The model under review builds one solid part; all positions refer to its coordinate system, in mm. A direction names the side the tool comes from. Round coordinates to 2 decimals unless told otherwise and drop trailing zeros. Order: outer loops, then holes, each group sorted by start corner. A loop starts at its lowest first (then second) coordinate and runs counter-clockwise, first axis right, second up. Notation, with made-up numbers: M -12,-27 L 10,-27 A16 ccw 10,-2 Z; hole C -28.5,38 d4. An arc over 180 degrees is marked long. Use a Markdown table: item, result. Add a question column.
1. The part is to be moulded in two halves that separate along X. For faces 4 (the cylindrical face through (0.04, -4.72, 1.76)), 5 (the cylindrical face through (-0.014, -4.393, -1.511)), say which applies: +X half, -X half, draft (parallel to the pull), parting line (faces both ways), or undercut.
2. Consider section A-A on y = 7. State the section outline as (x, z) points.
3. For faces 1 (the cylindrical face through (-0.108, 6.512, 0.004)), 2 (the flat face through (0.01, -3.3, -0.48)), 3 (the cylindrical face through (-0.192, -4.716, 0.048)), list the 3-axis set-ups (+Z, -Z, +X, -X, +Y, -Y) from which the entire face can be reached by the end or side of a thin tool; tool diameter is ignored.
4. Insertion check: P1, Ø2, axis at x = -2, y = 1.5, coming from the +Z side; P2, Ø1.5, axis at y = 4, z = -0.5, coming from the -X side; P3, Ø0.6, axis at x = -2.5, z = 0, coming from the +Y side. Each pin has a flat end and moves straight along its axis. Give the tip position at first contact, or say it passes through.
5. Consider section B-B on x = 0. State the section outline as (y, z) points.
6. To check wall thickness, follow probe 1 along Z at (x, y) = (-0.25, 5.5); probe 2 along X at (y, z) = (1.75, 0.1); probe 3 along Y at (x, z) = (0.5, 1.55). State the ranges of each line that lie inside material, in increasing order.
7. Consider section D-D on x = -0.75. State the section outline as (y, z) points, then the cut area to 3 significant figures.
8. Consider section C-C on z = 0.7. State the section outline as (x, y) points, then the cut area to 3 significant figures.
from build123d import *

# Parameters (mm, degrees)
MAINBODYS_W                           = 2.8
MAINBODYS_H                           = 0.5
MAIN_BODY_DEPTH                       = 9.5
BOTTOM_OF_MAIN_BODY_REACH             = 11.606
BOTTOM_OF_MAIN_BODY_DIRECTION_2_REACH = 11.606
TOPHOLES_R                            = 0.5
TOP_HOLE_DEPTH                        = 11.069260152
F_45_DEGREE_FLANGE_DEPTH              = 2
BOTTOM_FLAT_FLANGE_DEPTH              = 2
EXTENDEDBOTTOMFLANGES_W               = 2
EXTENDEDBOTTOMFLANGES_H               = 0.5
EXTENDED_BOTTOM_FLANGE_DEPTH          = 0.4
BOSSEDCYLINDERBODYS_R                 = 0.5
BOSSED_CYLINDER_BODY_DEPTH            = 0.5
C_MAIN_BODY_SIZE                      = 0.4


# Sheet-metal steps are written as plain solids
with BuildPart() as part:
    # MainBodyS → MAIN BODY (new body)
    with BuildSketch(Plane(origin=(0, 0, 0), x_dir=(1, 0, 0), z_dir=(0, 1, 0))):
        Rectangle(MAINBODYS_W, MAINBODYS_H)
    extrude(amount=MAIN_BODY_DEPTH)

    # BOTTOM OF MAIN BODY: up to this face of the body (flat: up to its plane)
    bottom_of_main_body_end = Plane(part.part.faces().sort_by_distance((0, 4.75, 0.25))[0])
    # BottomMainBodyS → BOTTOM OF MAIN BODY (add, up to the picked face)
    with BuildSketch(Plane.XY, mode=Mode.PRIVATE) as bottom_of_main_body_sk1:
        Polygon((0, 0), (2.8, 0), (2.8, -2), (3.3, -5), (2.2, -5), (1.2, -2.2), (0, -2.2), align=None)
    bottom_of_main_body_tool1 = split(extrude(bottom_of_main_body_sk1.sketch, amount=BOTTOM_OF_MAIN_BODY_REACH, mode=Mode.PRIVATE), bisect_by=bottom_of_main_body_end, keep=Keep.BOTH, mode=Mode.PRIVATE)
    bottom_of_main_body = bottom_of_main_body_tool1.solids().sort_by(Axis((1.768001, -2.02309, 0), (0, 0, 1)))[0]
    add(bottom_of_main_body)

    # BOTTOM OF MAIN BODY direction 2: up to this face of the body (flat: up to its plane)
    bottom_of_main_body_direction_2_end = Plane(part.part.faces().sort_by_distance((0, 4.75, -0.25))[0])
    # BottomMainBodyS → BOTTOM OF MAIN BODY direction 2 (add, up to the picked face)
    with BuildSketch(Plane.XY, mode=Mode.PRIVATE) as bottom_of_main_body_direction_2_sk1:
        Polygon((0, 0), (2.8, 0), (2.8, -2), (3.3, -5), (2.2, -5), (1.2, -2.2), (0, -2.2), align=None)
    bottom_of_main_body_direction_2_tool1 = split(extrude(bottom_of_main_body_direction_2_sk1.sketch, amount=-BOTTOM_OF_MAIN_BODY_DIRECTION_2_REACH, mode=Mode.PRIVATE), bisect_by=bottom_of_main_body_direction_2_end, keep=Keep.BOTH, mode=Mode.PRIVATE)
    bottom_of_main_body_direction_2 = bottom_of_main_body_direction_2_tool1.solids().sort_by(Axis((1.768001, -2.02309, 0), (0, 0, -1)))[0]
    add(bottom_of_main_body_direction_2)

    # BMB HM: BOTTOM OF MAIN BODY, BOTTOM OF MAIN BODY direction 2 across plane
    add(bottom_of_main_body.mirror(Plane(origin=(0, 0, 0), x_dir=(0, 0, 1), z_dir=(1, 0, 0))))
    add(bottom_of_main_body_direction_2.mirror(Plane(origin=(0, 0, 0), x_dir=(0, 0, 1), z_dir=(1, 0, 0))))

    # TopHoleS → TOP HOLE (cut, through all)
    with BuildSketch(Plane.XY.offset(0.25)):
        with Locations((0, 7)):
            Circle(TOPHOLES_R)
    extrude(amount=-TOP_HOLE_DEPTH, mode=Mode.SUBTRACT)

    # 45 DEGREE FLANGE section (across the edge) → 45 DEGREE FLANGE (add)
    with BuildSketch(Plane(origin=(1, -2.365685425, -0.25), x_dir=(0, 0.7071067811865438, -0.7071067811865512), z_dir=(-1, 0, 0))):
        with BuildLine():
            Line((-0.5, 0.165685425), (-0.5, 1.5))
            Line((-0.5, 1.5), (0, 1.5))
            Line((0, 1.5), (0, 0.165685425))
            ThreePointArc((0, 0.165685425), (0.030448187, 0.012612052), (0.117157288, -0.117157288))
            Line((0.117157288, -0.117157288), (-0.236396103, -0.470710678))
            ThreePointArc((-0.236396103, -0.470710678), (-0.431491579, -0.178729664), (-0.5, 0.165685425))
        make_face()
    extrude(amount=F_45_DEGREE_FLANGE_DEPTH)

    # BOTTOM FLAT FLANGE section (across the edge) → BOTTOM FLAT FLANGE (add)
    with BuildSketch(Plane(origin=(-1, -4.4627417, -1.639949494), x_dir=(0, 1, 0), z_dir=(1, 0, 0))):
        with BuildLine():
            Line((-0.5, 0.965685425), (-0.5, 1))
            Line((-0.5, 1), (0, 1))
            Line((0, 1), (0, 0.965685425))
            ThreePointArc((0, 0.965685425), (0.246926627, 0.596133612), (0.682842712, 0.682842712))
            Line((0.682842712, 0.682842712), (1.036396103, 0.329289322))
            ThreePointArc((1.036396103, 0.329289322), (0.055584911, 0.134193846), (-0.5, 0.965685425))
        make_face()
    extrude(amount=BOTTOM_FLAT_FLANGE_DEPTH)

    # ExtendedBottomFlangeS → EXTENDED BOTTOM FLANGE (add)
    with BuildSketch(Plane.XY.offset(-0.639949494)):
        with Locations((0, -4.7127417)):
            Rectangle(EXTENDEDBOTTOMFLANGES_W, EXTENDEDBOTTOMFLANGES_H)
    extrude(amount=EXTENDED_BOTTOM_FLANGE_DEPTH)

    # BossedCylinderBodyS → BOSSED  CYLINDER BODY (add)
    with BuildSketch(Plane.XZ.offset(4.9627417)):
        with BuildLine():
            Line((-1, -0.239949494), (1, -0.239949494))
            ThreePointArc((1, -0.239949494), (0, 1.760050506), (-1, -0.239949494))
        make_face()
        with Locations(Location((0, 0.510050506, 0), (0, 0, 270))):
            Circle(BOSSEDCYLINDERBODYS_R, mode=Mode.SUBTRACT)
    extrude(amount=-BOSSED_CYLINDER_BODY_DEPTH)

    # C MAIN BODY
    c_main_body_edges = [part.edges().sort_by_distance(p)[0] for p in [
        (-1.4, 9.5, 0),
        (1.4, 9.5, 0),
    ]]
    chamfer(c_main_body_edges, length=C_MAIN_BODY_SIZE)


solid = part.part
Answer block:
| question | item | result |
|---|---|---|
| 1 | face 4 | undercut |
| 1 | face 5 | draft |
| 2 | outline | M -1.4,-0.25 L -0.5,-0.25 L -0.5,0.25 L -1.4,0.25 Z; M 0.5,-0.25 L 1.4,-0.25 L 1.4,0.25 L 0.5,0.25 Z |
| 3 | face 1 | +Z, -Z |
| 3 | face 2 | +Z |
| 3 | face 3 | -Y |
| 4 | P1 | z = 0.25 |
| 4 | P2 | x = -1.4 |
| 4 | P3 | y = 0 |
| 5 | outline | M -4.96,-0.67 A0.9 ccw -3.43,-1.31 L -2.48,-0.37 A0.4 cw -2.2,-0.25 L 6.5,-0.25 L 6.5,0.25 L -2.2,0.25 A0.9 ccw -2.84,-0.01 L -3.78,-0.96 A0.4 cw -4.46,-0.67 L -4.46,0.01 L -4.96,0.01 Z; M -4.96,1.01 L -4.46,1.01 L -4.46,1.76 L -4.96,1.76 Z; M 7.5,-0.25 L 9.5,-0.25 L 9.5,0.25 L 7.5,0.25 Z |
| 6 | probe 1 | -0.25 to 0.25 |
| 6 | probe 2 | -1.4 to 1.4 |
| 6 | probe 3 | -4.96 to -4.46 |
| 7 | outline | M -4.96,-0.67 A0.9 ccw -3.43,-1.31 L -2.48,-0.37 A0.4 cw -2.2,-0.25 L 9.5,-0.25 L 9.5,0.25 L -2.2,0.25 A0.9 ccw -2.84,-0.01 L -3.78,-0.96 A0.4 cw -4.46,-0.67 L -4.46,1.51 L -4.96,1.51 Z |
| 7 | area | 8.63 mm^2 |
| 8 | outline | M -1.24,-4.96 L -0.46,-4.96 L -0.46,-4.46 L -1.24,-4.46 Z; M 0.46,-4.96 L 1.24,-4.96 L 1.24,-4.46 L 0.46,-4.46 Z |
| 8 | area | 0.773 mm^2 |
